Verification items for the finished model (mm, model axes). A direction names the side the tool comes from. Give positions to 0.01 mm unless a question says otherwise; leave off trailing zeros. Write each loop counter-clockwise with the first axis right and the second up, starting at its lowest first coordinate (ties: lowest second). Pieces come first, ordered by that corner, then holes. Notation, with made-up numbers: (-19, -15.5) - (11, -15.5) arc R16 ccw to (11, -10.5) - close; hole circle Ø10 at (50, 81.5). An arc over 180 degrees is marked (long way). Put each result on its own line as item: value.
from build123d import *

# Parameters (mm, degrees)
SKETCH_1_R               = 4
EXTRUDE_1_DEPTH          = 70.491679884
CUT_EXTRUDE_1_DEPTH      = 82.76843482
CUT_EXTRUDE_1_DEPTH_BACK = 82.76843482
SKETCH_2_R               = 1.6
CUT_EXTRUDE_START        = -82.76843482
SKETCH_3_W               = 3
SKETCH_3_H               = 5.6
CUT_EXTRUDE_2_DEPTH      = 150.536869639


with BuildPart() as part:
    # ｽｹｯﾁ1 → ﾎﾞｽ - 押し出し1 (new body)
    with BuildSketch(Plane.XY):
        with Locations(Location((2, 37, 0), (0, 0, 90))):
            Circle(SKETCH_1_R)
    extrude(amount=EXTRUDE_1_DEPTH)

    # ｽｹｯﾁ2 → ｶｯﾄ - 押し出し1 (cut, two sides: drawn at the far end of the back side and taken through both)
    with BuildSketch(Plane(origin=(0, 0, 0), x_dir=(-1, 0, 0), z_dir=(0, 0, -1)).offset(-CUT_EXTRUDE_1_DEPTH_BACK)):
        with Locations((-2, 37)):
            Circle(SKETCH_2_R)
    extrude(amount=CUT_EXTRUDE_1_DEPTH + CUT_EXTRUDE_1_DEPTH_BACK, mode=Mode.SUBTRACT)

    # ｽｹｯﾁ3 → ｶｯﾄ - 押し出し2 (cut)
    with BuildSketch(Plane(origin=(0, 0, 0), x_dir=(0, 0, -1), z_dir=(1, 0, 0)).offset(CUT_EXTRUDE_START)):
        with Locations((-4.5, 37)):
            Rectangle(SKETCH_3_W, SKETCH_3_H)
    cut_extrude_2 = extrude(amount=CUT_EXTRUDE_2_DEPTH, mode=Mode.SUBTRACT)

    # ﾐﾗｰ1: ｶｯﾄ - 押し出し2 across plane
    add(cut_extrude_2.mirror(Plane(origin=(0, 0, 35.245839942), x_dir=(1, 0, 0), z_dir=(0, 0, -1))), mode=Mode.SUBTRACT)


solid = part.part
Q1. Set-up check for faces 5 (the face through (2, 39.8, 66)), 6 (the face through (2, 39, 70.492)): record each of +Z, -Z, +X, -X, +Y, -Y from which the full face is reachable in a straight line by a thin tool's end or side.
Answers follow:
face 5: +X, -X
face 6: +Z, +X, -X, +Y, -Y
Q2. Scan lines: line 1 along Z through (x, y) = (4, 39.5); line 2 along X through (y, z) = (37, 1.05); line 3 along X through (y, z) = (36, 34). Record each from-to range of solid material in increasing order.
Answers follow:
line 1: z = 0 to 3, 6 to 64.49, 67.49 to 70.49
line 2: x = -2 to 0.4, 3.6 to 6
line 3: x = -1.87 to 0.75, 3.25 to 5.87
Q3. Go/stop test with flat-tipped pins: pin 1 Ø3 at (x, y) = (2, 37) entering from +Z; pin 2 Ø0.9 at (x, z) = (0.5, 5) entering from -Y; pin 3 Ø3 at (y, z) = (39, 17) entering from +X. Record where each tip stops, or that it passes through.
Answers follow:
pin 1: passes through
pin 2: stops at y = 33.14
pin 3: stops at x = 5.97
Q4. Section check B-B, the plane y = 37. Record the cut outline in (x, z), plus the area to 3 significant figures.
Answers follow:
outline: (-2, 0) - (0.4, 0) - (0.4, 3) - (-2, 3) - close; (-2, 6) - (0.4, 6) - (0.4, 64.49) - (-2, 64.49) - close; (-2, 67.49) - (0.4, 67.49) - (0.4, 70.49) - (-2, 70.49) - close; (3.6, 0) - (6, 0) - (6, 3) - (3.6, 3) - close; (3.6, 6) - (6, 6) - (6, 64.49) - (3.6, 64.49) - close; (3.6, 67.49) - (6, 67.49) - (6, 70.49) - (3.6, 70.49) - close
area: 310 mm2
Q5. Release check for a two-part mould opening along X. For faces 1 (the face through (2, 33, 35)), 2 (the face through (1.26, 35.58, 69.01)), 3 (the face through (2, 39, 0)), 4 (the face through (1.26, 35.58, 1.52)) record: released by +X, released by -X, zero draft, split by the parting line, or undercut.
Answers follow:
face 1: split by the parting line
face 2: undercut
face 3: zero draft
face 4: undercut
Q6. Section check C-C, the plane z = 8. Record the cut outline in (x, y).
Answers follow:
outline: circle Ø8 at (2, 37); hole circle Ø3.2 at (2, 37)
Q7. Section check A-A, the plane x = 2. Record the cut outline in (y, z), plus the area to 3 significant figures.
Answers follow:
outline: (33, 0) - (35.4, 0) - (35.4, 3) - (34.2, 3) - (34.2, 6) - (35.4, 6) - (35.4, 64.49) - (34.2, 64.49) - (34.2, 67.49) - (35.4, 67.49) - (35.4, 70.49) - (33, 70.49) - close; (38.6, 0) - (41, 0) - (41, 70.49) - (38.6, 70.49) - (38.6, 67.49) - (39.8, 67.49) - (39.8, 64.49) - (38.6, 64.49) - (38.6, 6) - (39.8, 6) - (39.8, 3) - (38.6, 3) - close
area: 324 mm2
